For this review, take the finished solid that the model builds, in its own axes (mm). A direction names the side the tool comes from. Coordinates: 2 decimals unless noted, no trailing zeros. Order: outer loops, then holes, each group sorted by start corner. A loop starts at its lowest first (then second) coordinate and runs counter-clockwise, first axis right, second up.
from build123d import *

# Parameters (mm, degrees)
BOSS_EXTRUDE1_DEPTH = 20
SKETCH2_W           = 19
SKETCH2_H           = 6
CUT_EXTRUDE1_DEPTH  = 20
SKETCH3_W           = 6
SKETCH3_H           = 19
CUT_EXTRUDE2_DEPTH  = 20
FILLET1_R           = 3


with BuildPart() as part:
    # Sketch1 → Boss-Extrude1 (new body)
    with BuildSketch(Plane.XY):
        Polygon((4, -20), (36, -20), (36, -12), (4, -12), (4, 20), (-4, 20), (-4, -20), align=None)
    extrude(amount=BOSS_EXTRUDE1_DEPTH)

    # Sketch2 → Cut-Extrude1 (cut)
    with BuildSketch(Plane(origin=(0, -12, 0), x_dir=(1, 0, 0), z_dir=(0, 1, 0))):
        with Locations((20, -10)):
            Rectangle(SKETCH2_W, SKETCH2_H)
    extrude(amount=-CUT_EXTRUDE1_DEPTH, mode=Mode.SUBTRACT)

    # Sketch3 → Cut-Extrude2 (cut)
    with BuildSketch(Plane(origin=(4, 0, 0), x_dir=(0, 0, -1), z_dir=(1, 0, 0))):
        with Locations((-10, 4)):
            Rectangle(SKETCH3_W, SKETCH3_H)
    extrude(amount=-CUT_EXTRUDE2_DEPTH, mode=Mode.SUBTRACT)

    # Fillet1
    fillet1_edges = [part.edges().sort_by_distance(p)[0] for p in [
        (29.5, -16, 7),
        (29.5, -16, 13),
        (10.5, -16, 7),
        (10.5, -16, 13),
        (0, -5.5, 13),
        (0, -5.5, 7),
        (0, 13.5, 13),
        (0, 13.5, 7),
    ]]
    fillet(fillet1_edges, radius=FILLET1_R - 0.0001)  # a hair under: the kernel refuses the full size


solid = part.part
1. The part is to be moulded in two halves that separate along X. For faces 1 (the face through (-4, 0, 5)), 2 (the face through (4, 4, 5)), 3 (the face through (11.4, -16.06, 12.14)), 4 (the face through (0, 4, 7)), say which applies: +X half, -X half, draft (parallel to the pull), parting line (faces both ways), or undercut.
Answer below:
face 1: -X half
face 2: +X half
face 3: undercut
face 4: draft
2. Take a section at A-A, the plane x = 14. Give the boundary of the cut face in (y, z).
Answer below:
outline: (-20, 0) - (-12, 0) - (-12, 7) - (-20, 7) - close; (-20, 13) - (-12, 13) - (-12, 20) - (-20, 20) - close
3. Clearance check with flat-ended pins moving along their axes: pin 1 Ø5 at (y, z) = (-6.5, 10.5) entering from +X; pin 2 Ø1.5 at (x, z) = (25.5, 10.5) entering from +Y; pin 3 Ø3 at (x, z) = (21, 14) entering from +Y. State where each tip first meets the part, or that it passes through.
Answer below:
pin 1: stops at x = 4
pin 2: passes through
pin 3: stops at y = -12
4. Machinability: for faces 5 (the face through (28.64, -16.06, 7.9)), 6 (the face through (20, -12, 5)), 7 (the face through (36, -16, 10)), 8 (the face through (-0.06, 12.64, 12.1)), 9 (the face through (0, 20, 10)), which of the approach directions +Z, -Z, +X, -X, +Y, -Y give a long, thin tool a straight path to every point of the face, cutting with its end or side? Answer none if there is none.
Answer below:
face 5: +Y, -Y
face 6: +Z, -Z, +X, +Y
face 7: +Z, -Z, +X, +Y, -Y
face 8: +X, -X
face 9: +Z, -Z, +X, -X, +Y
5. To check wall thickness, follow L1, parallel to Z at x = 3.5, y = -2; L2, parallel to X at y = -17, z = 10.25; L3, parallel to X at y = -9.5, z = 9.5. State the ranges of each line that lie inside material, in increasing order.
Answer below:
L1: z = 0 to 7, 13 to 20
L2: x = -4 to 10.51, 29.49 to 36
L3: x = -4 to 4
6. Take a section at B-B, the plane y = 4.5. Give the boundary of the cut face in (x, z), plus the area to 3 significant figures.
Answer below:
outline: (-4, 0) - (4, 0) - (4, 7) - (-4, 7) - close; (-4, 13) - (4, 13) - (4, 20) - (-4, 20) - close
area: 112 mm2
7. Take a section at C-C, the plane z = 10.75. Give the boundary of the cut face in (x, y), plus the area to 3 significant figures.
Answer below:
outline: (-4, -20) - (10.6, -20) - (10.6, -12) - (4, -12) - (4, -5.4) - (-4, -5.4) - close; (-4, 13.4) - (4, 13.4) - (4, 20) - (-4, 20) - close; (29.4, -20) - (36, -20) - (36, -12) - (29.4, -12) - close
area: 275 mm2
